```python
from build123d import *

# Parameters (mm, degrees)
BOSS_EXTRUDE2_DEPTH = 35
FILLET1_R           = 0.5


with BuildPart() as part:
    # Sketch1 → Boss-Extrude2 (new body)
    # profile 1 of 16: a face of its own
    with BuildSketch(Plane(origin=(0, 0, 0), x_dir=(1, 0, 0), z_dir=(0, 1, 0))):
        with BuildLine():
            Line((-0.682874368, 2.6638661), (-0.958491781, 2.577555723))
            ThreePointArc((-0.958491781, 2.577555723), (-1.18434287, 2.481900878), (-1.400772687, 2.36650288))
            ThreePointArc((-1.400772687, 2.36650288), (-1.944543648, 1.944543648), (-2.36650288, 1.400772687))
            ThreePointArc((-2.36650288, 1.400772687), (-2.55302024, 1.02205071), (-2.679372725, 0.619242926))
            ThreePointArc((-2.679372725, 0.619242926), (-2.749220106, -0.065488988), (-2.646848542, -0.746118487))
            ThreePointArc((-2.646848542, -0.746118487), (-2.527956912, -1.082558936), (-2.36650288, -1.400772687))
            ThreePointArc((-2.36650288, -1.400772687), (-1.944543648, -1.944543648), (-1.400772687, -2.36650288))
            ThreePointArc((-1.400772687, -2.36650288), (-1.052379439, -2.540668714), (-0.682874368, -2.6638661))
            ThreePointArc((-0.682874368, -2.6638661), (0, -2.75), (0.682874368, -2.6638661))
            ThreePointArc((0.682874368, -2.6638661), (1.082558936, -2.527956912), (1.456731751, -2.332473495))
            ThreePointArc((1.456731751, -2.332473495), (1.990299888, -1.897684472), (2.399189994, -1.344019111))
            ThreePointArc((2.399189994, -1.344019111), (2.55302024, -1.02205071), (2.6638661, -0.682874368))
            ThreePointArc((2.6638661, -0.682874368), (2.728381551, -0.344142576), (2.75, 0))
            ThreePointArc((2.75, 0), (2.728381551, 0.344142576), (2.6638661, 0.682874368))
            ThreePointArc((2.6638661, 0.682874368), (2.527956912, 1.082558936), (2.332473495, 1.456731751))
            ThreePointArc((2.332473495, 1.456731751), (1.897684472, 1.990299888), (1.344019111, 2.399189994))
            ThreePointArc((1.344019111, 2.399189994), (1.02205071, 2.55302024), (0.682874368, 2.6638661))
            ThreePointArc((0.682874368, 2.6638661), (0, 2.75), (-0.682874368, 2.6638661))
        make_face()
        with BuildLine():
            ThreePointArc((-0.958491781, 2.200293959), (-0.065885125, 2.399095486), (0.836287098, 2.249583048))
            ThreePointArc((0.836287098, 2.249583048), (1.697056275, 1.697056275), (2.249583048, 0.836287098))
            ThreePointArc((2.249583048, 0.836287098), (2.362096454, 0.424853319), (2.4, 0))
            ThreePointArc((2.4, 0), (2.349543094, -0.489537791), (2.200293959, -0.958491781))
            ThreePointArc((2.200293959, -0.958491781), (1.649828868, -1.743004505), (0.836287098, -2.249583048))
            ThreePointArc((0.836287098, -2.249583048), (-0.065885125, -2.399095486), (-0.958491781, -2.200293959))
            ThreePointArc((-0.958491781, -2.200293959), (-1.723234871, -1.670467473), (-2.229029582, -0.889621899))
            ThreePointArc((-2.229029582, -0.889621899), (-2.399984108, 0.008733954), (-2.222495654, 0.905821764))
            ThreePointArc((-2.222495654, 0.905821764), (-1.717144383, 1.676727518), (-0.958491781, 2.200293959))
        make_face(mode=Mode.SUBTRACT)
    # profile 2 of 16: a face of its own
    with BuildSketch(Plane(origin=(0, 0, 0), x_dir=(1, 0, 0), z_dir=(0, 1, 0))):
        with BuildLine():
            Line((-0.927656245, 0.905821764), (-0.958491781, 2.200293959))
            ThreePointArc((-0.958491781, 2.200293959), (-1.717144383, 1.676727518), (-2.222495654, 0.905821764))
            Line((-2.222495654, 0.905821764), (-0.927656245, 0.905821764))
        make_face()
    # profile 3 of 16: a face of its own
    with BuildSketch(Plane(origin=(0, 0, 0), x_dir=(1, 0, 0), z_dir=(0, 1, 0))):
        with BuildLine():
            Line((-2.229029582, -0.889621899), (-2.222495654, 0.905821764))
            ThreePointArc((-2.222495654, 0.905821764), (-2.399984108, 0.008733954), (-2.229029582, -0.889621899))
        make_face()
    # profile 4 of 16: a face of its own
    with BuildSketch(Plane(origin=(0, 0, 0), x_dir=(1, 0, 0), z_dir=(0, 1, 0))):
        with BuildLine():
            Line((-0.958491781, -0.889621899), (-2.229029582, -0.889621899))
            ThreePointArc((-2.229029582, -0.889621899), (-1.723234871, -1.670467473), (-0.958491781, -2.200293959))
            Line((-0.958491781, -2.200293959), (-0.958491781, -0.889621899))
        make_face()
    # profile 5 of 16: a face of its own
    with BuildSketch(Plane(origin=(0, 0, 0), x_dir=(1, 0, 0), z_dir=(0, 1, 0))):
        with BuildLine():
            ThreePointArc((-0.958491781, -2.200293959), (-0.065885125, -2.399095486), (0.836287098, -2.249583048))
            Line((0.836287098, -2.249583048), (-0.958491781, -2.200293959))
        make_face()
    # profile 6 of 16: a face of its own
    with BuildSketch(Plane(origin=(0, 0, 0), x_dir=(1, 0, 0), z_dir=(0, 1, 0))):
        with BuildLine():
            ThreePointArc((0.836287098, -2.249583048), (1.649828868, -1.743004505), (2.200293959, -0.958491781))
            Line((2.200293959, -0.958491781), (0.836287098, -0.958491781))
            Line((0.836287098, -0.958491781), (0.836287098, -2.249583048))
        make_face()
    # profile 7 of 16: a face of its own
    with BuildSketch(Plane(origin=(0, 0, 0), x_dir=(1, 0, 0), z_dir=(0, 1, 0))):
        with BuildLine():
            ThreePointArc((2.4, 0), (2.362096454, 0.424853319), (2.249583048, 0.836287098))
            Line((2.249583048, 0.836287098), (2.200293959, -0.958491781))
            ThreePointArc((2.200293959, -0.958491781), (2.349543094, -0.489537791), (2.4, 0))
        make_face()
    # profile 8 of 16: a face of its own
    with BuildSketch(Plane(origin=(0, 0, 0), x_dir=(1, 0, 0), z_dir=(0, 1, 0))):
        with BuildLine():
            ThreePointArc((2.249583048, 0.836287098), (1.697056275, 1.697056275), (0.836287098, 2.249583048))
            Line((0.836287098, 2.249583048), (0.836287098, 0.905821764))
            Line((0.836287098, 0.905821764), (2.249583048, 0.836287098))
        make_face()
    # profile 9 of 16: a face of its own
    with BuildSketch(Plane(origin=(0, 0, 0), x_dir=(1, 0, 0), z_dir=(0, 1, 0))):
        with BuildLine():
            ThreePointArc((-2.646848542, -0.746118487), (-2.749220106, -0.065488988), (-2.679372725, 0.619242926))
            Line((-2.679372725, 0.619242926), (-3.931143789, 0.589424572))
            Line((-3.931143789, 0.589424572), (-5, -0.059543887))
            Line((-5, -0.059543887), (-3.901275064, -0.664461024))
            Line((-3.901275064, -0.664461024), (-2.646848542, -0.746118487))
        make_face()
    # profile 10 of 16: a face of its own
    with BuildSketch(Plane(origin=(0, 0, 0), x_dir=(1, 0, 0), z_dir=(0, 1, 0))):
        with BuildLine():
            ThreePointArc((-1.400772687, -2.36650288), (-1.944543648, -1.944543648), (-2.36650288, -1.400772687))
            Line((-2.36650288, -1.400772687), (-3.251889781, -2.286159588))
            Line((-3.251889781, -2.286159588), (-3.577637792, -3.49343002))
            Line((-3.577637792, -3.49343002), (-2.365007256, -3.173042114))
            Line((-2.365007256, -3.173042114), (-1.400772687, -2.36650288))
        make_face()
    # profile 11 of 16: a face of its own
    with BuildSketch(Plane(origin=(0, 0, 0), x_dir=(1, 0, 0), z_dir=(0, 1, 0))):
        with BuildLine():
            ThreePointArc((0.682874368, -2.6638661), (0, -2.75), (-0.682874368, -2.6638661))
            Line((-0.682874368, -2.6638661), (-0.682874368, -3.915992264))
            Line((-0.682874368, -3.915992264), (-0.059543887, -5))
            Line((-0.059543887, -5), (0.571366928, -3.915992264))
            Line((0.571366928, -3.915992264), (0.682874368, -2.6638661))
        make_face()
    # profile 12 of 16: a face of its own
    with BuildSketch(Plane(origin=(0, 0, 0), x_dir=(1, 0, 0), z_dir=(0, 1, 0))):
        with BuildLine():
            Line((3.305410563, -2.208070158), (2.399189994, -1.344019111))
            ThreePointArc((2.399189994, -1.344019111), (1.990299888, -1.897684472), (1.456731751, -2.332473495))
            Line((1.456731751, -2.332473495), (2.439899933, -3.115821544))
            Line((2.439899933, -3.115821544), (3.659816345, -3.407240789))
            Line((3.659816345, -3.407240789), (3.305410563, -2.208070158))
        make_face()
    # profile 13 of 16: a face of its own
    with BuildSketch(Plane(origin=(0, 0, 0), x_dir=(1, 0, 0), z_dir=(0, 1, 0))):
        with BuildLine():
            Line((3.915992264, 0.571366928), (2.6638661, 0.682874368))
            ThreePointArc((2.6638661, 0.682874368), (2.728381551, 0.344142576), (2.75, 0))
            ThreePointArc((2.75, 0), (2.728381551, -0.344142576), (2.6638661, -0.682874368))
            Line((2.6638661, -0.682874368), (3.915992264, -0.682874368))
            Line((3.915992264, -0.682874368), (5, -0.059543887))
            Line((5, -0.059543887), (3.915992264, 0.571366928))
        make_face()
    # profile 14 of 16: a face of its own
    with BuildSketch(Plane(origin=(0, 0, 0), x_dir=(1, 0, 0), z_dir=(0, 1, 0))):
        with BuildLine():
            Line((2.208070158, 3.305410563), (1.344019111, 2.399189994))
            ThreePointArc((1.344019111, 2.399189994), (1.897684472, 1.990299888), (2.332473495, 1.456731751))
            Line((2.332473495, 1.456731751), (3.115821544, 2.439899933))
            Line((3.115821544, 2.439899933), (3.407240789, 3.659816345))
            Line((3.407240789, 3.659816345), (2.208070158, 3.305410563))
        make_face()
    # profile 15 of 16: a face of its own
    with BuildSketch(Plane(origin=(0, 0, 0), x_dir=(1, 0, 0), z_dir=(0, 1, 0))):
        with BuildLine():
            Line((-0.682874368, 3.915992264), (-0.682874368, 2.6638661))
            ThreePointArc((-0.682874368, 2.6638661), (0, 2.75), (0.682874368, 2.6638661))
            Line((0.682874368, 2.6638661), (0.571366928, 3.915992264))
            Line((0.571366928, 3.915992264), (-0.059543887, 5))
            Line((-0.059543887, 5), (-0.682874368, 3.915992264))
        make_face()
    # profile 16 of 16: a face of its own
    with BuildSketch(Plane(origin=(0, 0, 0), x_dir=(1, 0, 0), z_dir=(0, 1, 0))):
        with BuildLine():
            ThreePointArc((-2.36650288, 1.400772687), (-1.944543648, 1.944543648), (-1.400772687, 2.36650288))
            Line((-1.400772687, 2.36650288), (-2.365007256, 3.173042114))
            Line((-2.365007256, 3.173042114), (-3.577637792, 3.49343002))
            Line((-3.577637792, 3.49343002), (-3.251889781, 2.286159588))
            Line((-3.251889781, 2.286159588), (-2.36650288, 1.400772687))
        make_face()
    extrude(amount=BOSS_EXTRUDE2_DEPTH)

    # Fillet1
    fillet1_edges = [part.edges().sort_by_distance(p)[0] for p in [
        (0.836287098, 17.5, -0.905821764),
        (-0.927656245, 17.5, -0.905821764),
        (-0.958491781, 17.5, 0.889621899),
        (0.836287098, 17.5, 0.958491781),
    ]]
    fillet(fillet1_edges, radius=FILLET1_R)


solid = part.part
```
For this review, take the finished solid that the model builds, in its own axes (mm). A direction names the side the tool comes from. Coordinates: 2 decimals unless noted, no trailing zeros. Write each loop counter-clockwise with the first axis right and the second up, starting at its lowest first coordinate (ties: lowest second). Pieces come first, ordered by that corner, then holes. Notation, with made-up numbers: (-4.5, 87.25) - (47.5, 87.25) arc R13 cw to (47.5, 101.25) - close; hole circle Ø6 at (41, 69.25). An arc over 180 degrees is marked (long way). Answer in a Markdown table with one row per item. Add a question column.
Q1. We need section A-A, the plane z = -4.5. State the section outline as (x, y) points.
Q2. For probe 1 along X at (y, z) = (11, -2.75); probe 2 along X at (y, z) = (29, 3); probe 3 along Z at (x, y) = (2.5, 12), list the stretches that pass through material, from the lowest coordinate up.
Q3. Draft analysis for pull direction X (two halves, no side actions). For faces 1 (the flat face through (3, 17, 0.683)), 2 (the flat face through (-1.876, 17.255, -2.764)), 3 (the flat face through (3.26, 17.26, -3.04)), 4 (the flat face through (-4.46, 17.26, -0.27)), state which applies: +X half, -X half, draft (parallel to the pull), parting line (faces both ways), or undercut.
Q4. Tool access review of faces 5 (the cylindrical face through (-0.08, 17.26, -2.4)), 6 (the flat face through (3.299, 17.255, -0.626)), 7 (the flat face through (0.626, 17.255, 3.299)): name each direction out of +Z, -Z, +X, -X, +Y, -Y from which nothing blocks a thin tool from reaching the whole face with its end or side.
Q5. For P1, Ø0.9, axis at y = 11, z = 2, coming from the -X side; P2, Ø0.6, axis at y = 9, z = 1.5, coming from the +X side; P3, Ø1.4, axis at y = 19.5, z = 3.5, coming from the -X side; P4, Ø5, axis at x = -3, z = 3.5, coming from the +Y side, all flat-tipped, find the tip position at first contact; note any pin that passes through.
Answer list:
| question | item | result |
|---|---|---|
| 1 | outline | (-0.35, 0) - (0.23, 0) - (0.23, 35) - (-0.35, 35) - close |
| 2 | probe 1 | x = -3.38 to -1.86, -0.68 to 0.68, 1.68 to 3.19 |
| 2 | probe 2 | x = -3.44 to -2.16, -0.68 to 0.65, 2.29 to 3.54 |
| 2 | probe 3 | z = -3.39 to -1.67, -1.15 to 1.15, 1.44 to 3.13 |
| 3 | face 1 | draft |
| 3 | face 2 | undercut |
| 3 | face 3 | +X half |
| 3 | face 4 | -X half |
| 4 | face 5 | +Y, -Y |
| 4 | face 6 | +X, +Y, -Y |
| 4 | face 7 | +Z, +Y, -Y |
| 5 | P1 | stops at x = -3.3 |
| 5 | P2 | stops at x = 2.88 |
| 5 | P3 | stops at x = -3.58 |
| 5 | P4 | stops at y = 35 |
